Could you check a few things on this model? Use its own coordinates, in mm. Coordinates: 2 decimals unless noted, no trailing zeros. Loops run counter-clockwise (first coordinate to the right, second up) from the corner with the lowest first, then second, coordinate; pieces in that order, holes last.
from build123d import *

# Parameters (mm, degrees)
SKETCH1_R                       = 10
BOSS_EXTRUDE1_DEPTH             = 10
M10_CLEARANCE_HOLE1_D           = 11
M10_CLEARANCE_HOLE1_ON_FACE_2_D = 11


with BuildPart() as part:
    # Sketch1 → Boss-Extrude1 (new body)
    with BuildSketch(Plane(origin=(0, 0, 0), x_dir=(0, 0, -1), z_dir=(1, 0, 0))):
        with BuildLine():
            ThreePointArc((-10, 50), (-11.202983752, 27.492262307), (-14.092449523, 5.138371963))
            ThreePointArc((-14.092449523, 5.138371963), (0, 15), (14.092449523, 5.138371963))
            ThreePointArc((14.092449523, 5.138371963), (11.202983752, 27.492262307), (10, 50))
            ThreePointArc((10, 50), (0, 40), (-10, 50))
        make_face()
        with Locations((0, 50)):
            Circle(SKETCH1_R)
        with BuildLine():
            ThreePointArc((-14.092449523, 5.138371963), (-14.535053081, 2.567212815), (-15, 0))
            ThreePointArc((-15, 0), (0, -15), (15, 0))
            ThreePointArc((15, 0), (14.535053081, 2.567212815), (14.092449523, 5.138371963))
            ThreePointArc((14.092449523, 5.138371963), (0, 15), (-14.092449523, 5.138371963))
        make_face()
    extrude(amount=BOSS_EXTRUDE1_DEPTH)

    # M10 Clearance Hole1 (through all)
    with Locations(Plane(origin=(10, 50, 0), x_dir=(0, 0, 1), z_dir=(1, 0, 0))):
        with Locations((0, 0), (0, 50)):
            Hole(M10_CLEARANCE_HOLE1_D / 2)

    # M10 Clearance Hole1 on face 2 (through all)
    with Locations(Plane(origin=(0, 0, 0), x_dir=(0, 0, -1), z_dir=(-1, 0, 0))):
        with Locations((0, 0)):
            Hole(M10_CLEARANCE_HOLE1_ON_FACE_2_D / 2)


solid = part.part
(1) For pin 1 (5 mm diameter, centred on x = 5, y = 44.5, fed in from +Z); pin 2 (6.5 mm diameter, centred on y = 50, z = 0, fed in from +X); pin 3 (4 mm diameter, centred on x = 8, y = 15, fed in from +Z); pin 4 (3 mm diameter, centred on x = 6, y = 41.5, fed in from -Z), each with a flat end and sliding along its axis, tell me the tip position at first contact or that it passes through.
Answers:
pin 1: stops at z = 10.23
pin 2: passes through
pin 3: stops at z = 12.88
pin 4: stops at z = -10.33
(2) Imagine slicing it at C-C, the plane y = 38. Write out the boundary of the cut face in (x, z), and give its area (3 significant figures).
Answers:
outline: (0, -10.43) - (10, -10.43) - (10, 10.43) - (0, 10.43) - close
area: 209 mm2
(3) Imagine slicing it at A-A, the plane z = 0. Write out the boundary of the cut face in (x, y), and give its area (3 significant figures).
Answers:
outline: (0, -15) - (10, -15) - (10, -5.5) - (0, -5.5) - close; (0, 5.5) - (10, 5.5) - (10, 44.5) - (0, 44.5) - close; (0, 55.5) - (10, 55.5) - (10, 60) - (0, 60) - close
area: 530 mm2
(4) We'd pull the mould along Y, two halves only. Please class faces 1 (the face through (4.93, 2.53, -14.54)), 2 (the face through (5, -15, 0)), 3 (the face through (4.93, 5.37, 1.19)): +Y half, -Y half, draft (parallel to the pull), parting line (faces both ways), or undercut.
Answers:
face 1: +Y half
face 2: -Y half
face 3: undercut
(5) I need wall thicknesses on probe 1 along Y at (x, z) = (3, 0); probe 2 along Z at (x, y) = (5.75, 50); probe 3 along Y at (x, z) = (3.75, 4). Which ranges of each line are inside material? Lowest first, please.
Answers:
probe 1: y = -15 to -5.5, 5.5 to 44.5, 55.5 to 60
probe 2: z = -10 to -5.5, 5.5 to 10
probe 3: y = -14.46 to -3.77, 3.77 to 46.23, 53.77 to 59.17
(6) Imagine slicing it at B-B, the plane x = 5. Write out the boundary of the cut face in (y, z).
Answers:
outline: (0, -15) arc R300 cw to (5.14, -14.09) arc R300 cw to (50, -10) arc R10 ccw to (50, 10) arc R300 cw to (5.14, 14.09) arc R300 cw to (0, 15) arc R15 ccw to start; hole circle Ø11 at (0, 0); hole circle Ø11 at (50, 0)
(7) Imagine slicing it at D-D, the plane z = -12. Write out the boundary of the cut face in (x, y), and give its area (3 significant figures).
Answers:
outline: (0, -9) - (10, -9) - (10, 19.84) - (0, 19.84) - close
area: 288 mm2
